Verification items for this drawing (mm, ordinates from the low corner). Coordinates: 2 decimals unless noted, no trailing zeros. Order: outer loops, then holes, each group sorted by start corner. A loop starts at its lowest first (then second) coordinate and runs counter-clockwise, first axis right, second up. Notation, with made-up numbers: M -39,80.25 L 16,80.25 A32 ccw 16,118.25 Z; hole C 43,-11.75 d10. An arc over 180 degrees is marked long. Return JSON: item names as keys, results as strings. Group by question number.
1. Mould release check, pull along Z, two halves, no side actions. Record for the marked faces 1, 2, 3 and 4: +Z half, -Z half, draft (parallel to the pull), parting line (faces both ways), or undercut.
2. Material ranges on line 1 along Z through (x, y) = (16, 3.25); line 2 along Y through (x, z) = (18.25, 10.5); line 3 along Z through (x, y) = (21.75, 0.5) (3 decimals), recorded low to high.
3. Gauge pin test, flat ends, axial feed: pin 1 (0.6 mm diameter, centred on x = 13, z = 34.5, fed in from -Y); pin 2 (2 mm diameter, centred on x = 19.5, y = 2.5, fed in from +Z); pin 3 (2 mm diameter, centred on x = 11.5, y = 3, fed in from -Z); pin 4 (1 mm diameter, centred on x = 15.5, z = 11, fed in from -Y). Record the tip position at first contact, or that the pin passes through.
4. Section check B-B, the plane y = 3.75. Record the cut outline in (x, z), plus the area to 3 significant figures.
5. Section check D-D, the plane y = 0.5. Record the cut outline in (x, z) (3 decimals), plus the area to 3 significant figures.
6. Section check C-C, the plane x = 10. Record the cut outline in (y, z), plus the area to 3 significant figures.
7. Section check A-A, the plane x = 22.5. Record the cut outline in (y, z) (3 decimals).
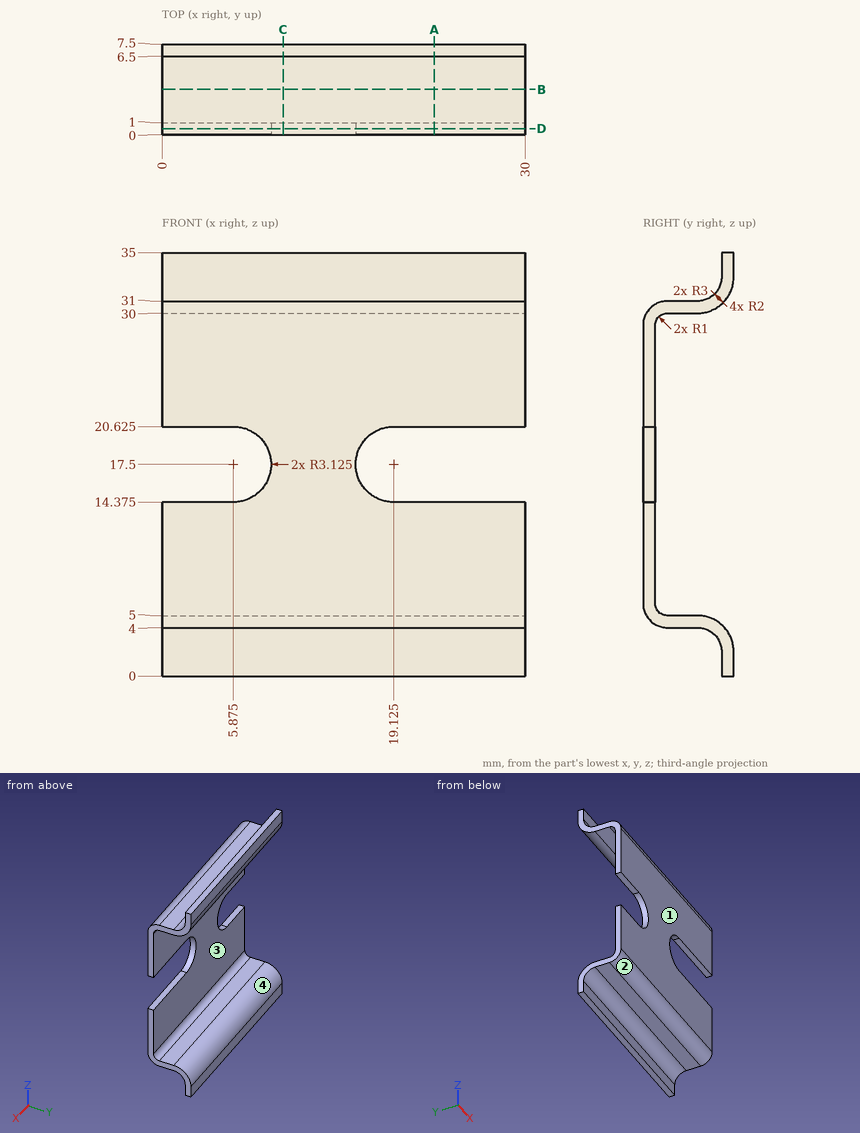
Answers follow:
{
 "1": {"face 1": "draft", "face 2": "-Z half", "face 3": "undercut", "face 4": "undercut"},
 "2": {"line 1": "4 to 5, 30 to 31", "line 2": "0 to 1", "line 3": "4.677 to 14.375, 20.625 to 30.323"},
 "3": {"pin 1": "y = 6.5", "pin 2": "z = 31", "pin 3": "z = 4", "pin 4": "y = 0"},
 "4": {"outline": "M 0,4 L 30,4 L 30,5 L 0,5 Z; M 0,30 L 30,30 L 30,31 L 0,31 Z", "area": "60.0 mm^2"},
 "5": {"outline": "M 0,4.677 L 30,4.677 L 30,14.375 L 19.125,14.375 A3.125 cw 19.125,20.625 L 30,20.625 L 30,30.323 L 0,30.323 L 0,20.625 L 5.875,20.625 A3.125 cw 5.875,14.375 L 0,14.375 Z", "area": "634 mm^2"},
 "6": {"outline": "M 0,6 A2 ccw 2,4 L 4.5,4 A2 cw 6.5,2 L 6.5,0 L 7.5,0 L 7.5,2 A3 ccw 4.5,5 L 2,5 A1 cw 1,6 L 1,29 A1 cw 2,30 L 4.5,30 A3 ccw 7.5,33 L 7.5,35 L 6.5,35 L 6.5,33 A2 cw 4.5,31 L 2,31 A2 ccw 0,29 Z", "area": "44.6 mm^2"},
 "7": {"outline": "M 0,6 A2 ccw 2,4 L 4.5,4 A2 cw 6.5,2 L 6.5,0 L 7.5,0 L 7.5,2 A3 ccw 4.5,5 L 2,5 A1 cw 1,6 L 1,14.375 L 0,14.375 Z; M 0,20.625 L 1,20.625 L 1,29 A1 cw 2,30 L 4.5,30 A3 ccw 7.5,33 L 7.5,35 L 6.5,35 L 6.5,33 A2 cw 4.5,31 L 2,31 A2 ccw 0,29 Z"}
}
